For this review, take the finished solid that the model builds, in its own axes (mm). Face numbers are marked on the shaded views. A direction names the side the tool comes from. Give positions to 0.01 mm unless a question says otherwise; leave off trailing zeros. Order: outer loops, then holes, each group sorted by start corner. A loop starts at its lowest first (then second) coordinate and runs counter-clockwise, first axis right, second up. Notation, with made-up numbers: M 79,46.5 L 94,46.5 A22 cw 94,71.5 Z; hole C 55,73.5 d8. An arc over 180 degrees is marked long. Use CSV: the item, a comma, the result in double quotes. Start each with the question number.
(1) Consider section A-A (z = -1.5). Write out the cut boundary in (x, y).
(2) Wall thickness on L1, parallel to X at y = -2.25, z = 0; L2, parallel to Z at x = 0, y = -1.3; L3, parallel to X at y = -0.9, z = 0: over which ranges is each line inside the solid? List them lowest first. Write a range as from..to.
(3) Clearance check with flat-ended pins moving along their axes: P1, Ø4, axis at x = -0.5, z = 2, coming from the -Y side; P2, Ø1.5, axis at y = -4, z = 1, coming from the -X side (3 decimals); P3, Ø0.8, axis at y = -1, z = 2, coming from the +X side; P4, Ø0.8, axis at x = -4, z = -2, coming from the +Y side. State where each tip first meets the part, or that it passes through.
(4) Consider section D-D (z = 3.25). Write out the cut boundary in (x, y).
(5) Draft analysis for pull direction Z (two halves, no side actions). For the marked faces 1, 2 and 3, state which applies: pulls with the +Z half, pulls with the -Z half, needs draft (parallel to the pull), parting line crosses it, or undercut.
(6) Tool access review of the marked faces 4, 5 and 6: name each direction out of +Z, -Z, +X, -X, +Y, -Y from which nothing blocks a thin tool from reaching the whole face with its end or side.
(7) Consider section C-C (x = 0). Write out the cut boundary in (y, z).
(8) Consider section B-B (y = -2). Write out the cut boundary in (x, z), and give its area (3 significant figures).
```python
from build123d import *

# Parameters (mm, degrees)
EXTRUDE_1_DEPTH     = 5
SKETCH_2_R          = 2.5
CUT_EXTRUDE_1_DEPTH = 5.5


with BuildPart() as part:
    # Эскиз1 → Бобышка-Вытянуть1 (new body, symmetric)
    with BuildSketch(Plane.XY):
        Polygon((3, 0), (-3, 0), (-3, -1.5), (-4.7, -1.5), (-4.7, -2.5), (-2.5, -4.5), (2.5, -4.5), (4.7, -2.5), (4.7, -1.5), (3, -1.5), align=None)
    extrude(amount=EXTRUDE_1_DEPTH, both=True)

    # Эскиз2 → Вырез-Вытянуть1 (cut, through all)
    with BuildSketch(Plane(origin=(0, 0, 0), x_dir=(1, 0, 0), z_dir=(0, 1, 0))):
        with Locations(Location((0, 0, 0), (0, 0, 270))):  # turned: the seam where the file's is
            Circle(SKETCH_2_R)
    extrude(amount=-CUT_EXTRUDE_1_DEPTH, mode=Mode.SUBTRACT)


solid = part.part
```
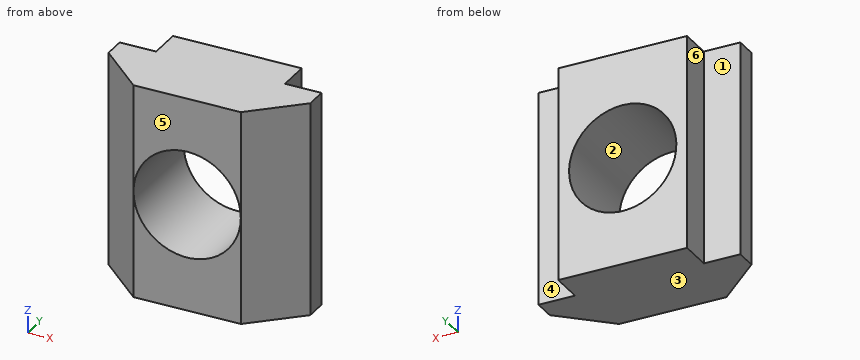
Check result:
1,outline,"M -4.7,-2.5 L -2.5,-4.5 L -2,-4.5 L -2,0 L -3,0 L -3,-1.5 L -4.7,-1.5 Z; M 2,-4.5 L 2.5,-4.5 L 4.7,-2.5 L 4.7,-1.5 L 3,-1.5 L 3,0 L 2,0 Z"
2,L1,"x = -4.7..-2.5, 2.5..4.7"
2,L2,"z = -5..-2.5, 2.5..5"
2,L3,"x = -3..-2.5, 2.5..3"
3,P1,"stops at y = -4.5"
3,P2,"stops at x = -3.875"
3,P3,"stops at x = 3"
3,P4,"stops at y = -1.5"
4,outline,"M -4.7,-2.5 L -2.5,-4.5 L 2.5,-4.5 L 4.7,-2.5 L 4.7,-1.5 L 3,-1.5 L 3,0 L -3,0 L -3,-1.5 L -4.7,-1.5 Z"
5,face 1,"needs draft"
5,face 2,"undercut"
5,face 3,"pulls with the -Z half"
6,face 4,"+Z, -Z, +X, +Y"
6,face 5,"+Z, -Z, +X, -X, -Y"
6,face 6,"+Z, -Z, -X, +Y"
7,outline,"M -4.5,-5 L 0,-5 L 0,-2.5 L -4.5,-2.5 Z; M -4.5,2.5 L 0,2.5 L 0,5 L -4.5,5 Z"
8,outline,"M -4.7,-5 L 4.7,-5 L 4.7,5 L -4.7,5 Z; hole C 0,0 d5"
8,area,"74.4 mm^2"
